Geometry: final body of the model. Coordinates: model frame, mm. Face numbers are marked on the shaded views. Round coordinates to 2 decimals unless told otherwise and drop trailing zeros. Loops run counter-clockwise (first coordinate to the right, second up) from the corner with the lowest first, then second, coordinate; pieces in that order, holes last. Notation, with made-up numbers: M 14,-38 L 63,-38 A23 ccw 63,-5 Z; hole C 62.25,70.25 d8. An arc over 180 degrees is marked long. Return JSON: item names as keys, results as strings.
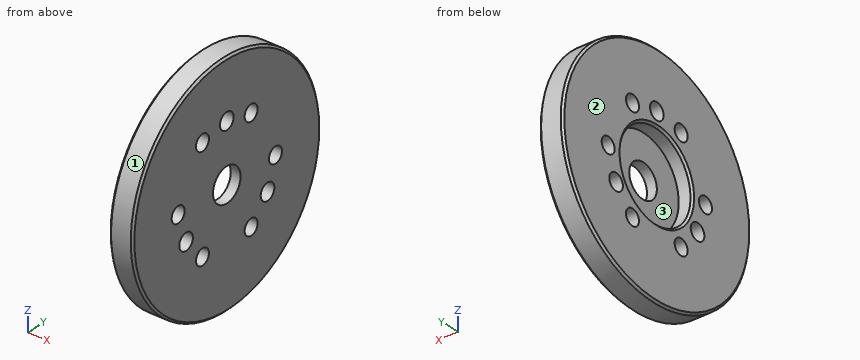
from build123d import *

# Parameters (mm, degrees)
F0_R     = 29
F0_R_2   = 2
F0_R_3   = 2.1
F0_R_4   = 4.25
F1_DEPTH = 6
F2_R     = 11
F3_DEPTH = 3.5
F4_SIZE  = 0.5


# Not quite as in the source:
# - a feature names something its author has since deleted; it is built from what else it names


with BuildPart() as f1:
    # F0 (on Right) → F1 (new body)
    with BuildSketch(Plane.YZ):
        Circle(F0_R)
        with Locations((-7.5, -12.9903810568)):
            Circle(F0_R_2, mode=Mode.SUBTRACT)
        with Locations((-12.5573683549, -7.25)):
            Circle(F0_R_3, mode=Mode.SUBTRACT)
        with Locations((7.5, -12.9903810568)):
            Circle(F0_R_2, mode=Mode.SUBTRACT)
        with Locations((12.5573683549, -7.25)):
            Circle(F0_R_3, mode=Mode.SUBTRACT)
        with Locations((-15, 0)):
            Circle(F0_R_2, mode=Mode.SUBTRACT)
        with Locations((-7.5, 12.9903810568)):
            Circle(F0_R_2, mode=Mode.SUBTRACT)
        Circle(F0_R_4, mode=Mode.SUBTRACT)
        with Locations((7.5, 12.9903810568)):
            Circle(F0_R_2, mode=Mode.SUBTRACT)
        with Locations((15, 0)):
            Circle(F0_R_2, mode=Mode.SUBTRACT)
        with Locations((0, 14.5)):
            Circle(F0_R_3, mode=Mode.SUBTRACT)
    extrude(amount=F1_DEPTH)

    # F2 (on Right) → F3 (cut)
    with BuildSketch(Plane.YZ):
        Circle(F2_R)
    extrude(amount=F3_DEPTH, mode=Mode.SUBTRACT)

    # F4
    f4_edges = [f1.edges().sort_by_distance(p)[0] for p in [
        (0, -11, 0),
        (0, -29, 0),
        (6, -29, 0),
    ]]
    chamfer(f4_edges, length=F4_SIZE)


solid = f1.part
Q1. Section query B-B (y = 0). Output: boundary loops of the cut face in (x, z).
Determined:
{"outline": "M 0,-28.5 L 0.5,-29 L 5.5,-29 L 6,-28.5 L 6,-4.25 L 3.5,-4.25 L 3.5,-11 L 0.5,-11 L 0,-11.5 Z; M 0,11.5 L 0.5,11 L 3.5,11 L 3.5,4.25 L 6,4.25 L 6,12.4 L 0,12.4 Z; M 0,16.6 L 6,16.6 L 6,28.5 L 5.5,29 L 0.5,29 L 0,28.5 Z"}
Q2. Pull-direction query (Y, two-part tool) for the marked faces 1, 2 and 3; classes: pulls with the +Y half, pulls with the -Y half, needs draft (parallel to the pull), parting line crosses it, or undercut.
Determined:
{"face 1": "parting line crosses it", "face 2": "needs draft", "face 3": "undercut"}
Q3. Section query C-C (x = 4.4). State how many separate pieces and enclosed holes the cut face has, plus the area to 3 significant figures.
Determined:
{"separate pieces": "1", "enclosed holes": "10", "area": "2,470 mm^2"}
Q4. Section query A-A (z = 0). Output: boundary loops of the cut face in (x, y), plus the area to 3 significant figures.
Determined:
{"outline": "M 0,-28.5 L 0.5,-29 L 5.5,-29 L 6,-28.5 L 6,-17 L 0,-17 Z; M 0,-13 L 6,-13 L 6,-4.25 L 3.5,-4.25 L 3.5,-11 L 0.5,-11 L 0,-11.5 Z; M 0,11.5 L 0.5,11 L 3.5,11 L 3.5,4.25 L 6,4.25 L 6,13 L 0,13 Z; M 0,17 L 6,17 L 6,28.5 L 5.5,29 L 0.5,29 L 0,28.5 Z", "area": "201 mm^2"}
Q5. Pin query (flat end, axial travel): pin 1 (3.5 mm diameter, centred on y = 12.56, z = -7.25, fed in from -X); pin 2 (17.5 mm diameter, centred on y = 0.5, z = 2.5, fed in from -X); pin 3 (2 mm diameter, centred on x = 2, y = 10, fed in from -Z); pin 4 (1 mm diameter, centred on x = 1, y = 2, fed in from +Z). Return the tip coordinate at first contact, or that it passes through.
Determined:
{"pin 1": "passes through", "pin 2": "stops at x = 0.2", "pin 3": "stops at z = -27.57", "pin 4": "stops at z = 28.96"}
Q6. Material intervals for L1, parallel to Z at x = 1.7, y = 0; L2, parallel to Z at x = 3.7, y = 0; L3, parallel to Y at x = 3.5, z = -14, sorted ascending.
Determined:
{"L1": "z = -29 to -11, 11 to 12.4, 16.6 to 29", "L2": "z = -29 to -4.25, 4.25 to 12.4, 16.6 to 29", "L3": "y = -25.4 to -9.23, -5.77 to 5.77, 9.23 to 25.4"}
